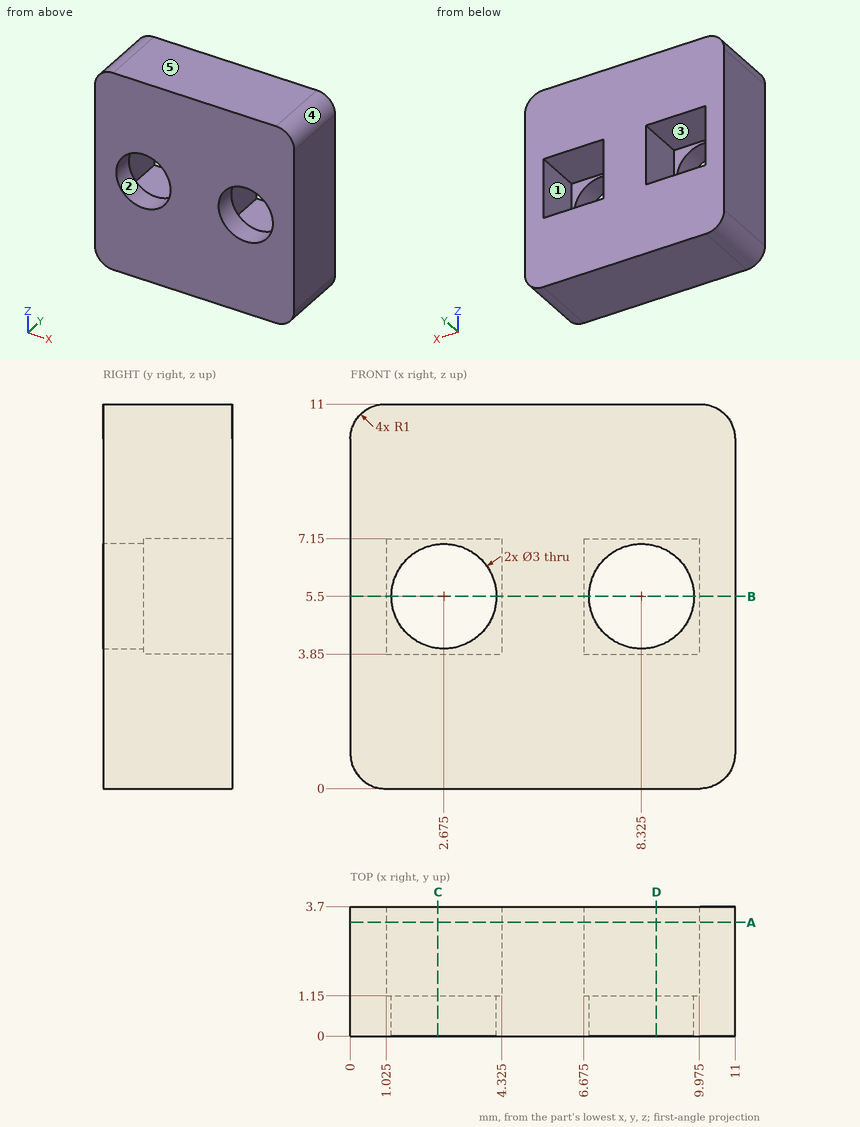
Drawing for the job (mm, zero at the part's lowest x, y, z). A direction names the side the tool comes from. Give positions to 0.01 mm unless a question says otherwise; leave off trailing zeros. Order: outer loops, then holes, each group sorted by start corner. A loop starts at its lowest first (then second) coordinate and runs counter-clockwise, first axis right, second up. Notation, with made-up numbers: M 73.5,-15.75 L 77.5,-15.75 A30 ccw 77.5,17.25 Z; hole C 77.5,57.25 d4. An arc over 180 degrees is marked long. Use a Markdown table: item, result. Add a question column.
(1) Saw through at D-D, the plane x = 8.75. Give the cut face in (y, z).
(2) Saw through at B-B, the plane z = 5.5. Give the cut face in (x, y) (3 decimals), and give its area (3 significant figures).
(3) 3-axis set-ups, long thin cutter, end or side, ignore diameter. For the marked faces 1 and 2: which of +Z, -Z, +X, -X, +Y, -Y reach the whole face in a straight line?
(4) Mould opens along X. For the marked faces 3, 4 and 5 say: +X half, -X half, draft (parallel to the pull), parting line (faces both ways), or undercut.
(5) Probe line 1 along X through (y, z) = (3, 4.25) (3 decimals); line 2 along X through (y, z) = (0.55, 5.5) (3 decimals); line 3 along Z through (x, y) = (4, 1.95). List the from-to ranges inside material, lowest first. Write a range as [from, to].
(6) Saw through at A-A, the plane y = 3.25. Give the cut face in (x, z) (3 decimals).
(7) Saw through at C-C, the plane x = 2.5. Give the cut face in (y, z).
Answer key:
| question | item | result |
|---|---|---|
| 1 | outline | M 0,0 L 3.7,0 L 3.7,3.85 L 1.15,3.85 L 1.15,4.06 L 0,4.06 Z; M 0,6.94 L 1.15,6.94 L 1.15,7.15 L 3.7,7.15 L 3.7,11 L 0,11 Z |
| 2 | outline | M 0,0 L 1.175,0 L 1.175,1.15 L 1.025,1.15 L 1.025,3.7 L 0,3.7 Z; M 4.175,0 L 6.825,0 L 6.825,1.15 L 6.675,1.15 L 6.675,3.7 L 4.325,3.7 L 4.325,1.15 L 4.175,1.15 Z; M 9.825,0 L 11,0 L 11,3.7 L 9.975,3.7 L 9.975,1.15 L 9.825,1.15 Z |
| 2 | area | 17.0 mm^2 |
| 3 | face 1 | +Y |
| 3 | face 2 | +Y, -Y |
| 4 | face 3 | undercut |
| 4 | face 4 | +X half |
| 4 | face 5 | draft |
| 5 | line 1 | [0, 1.025], [4.325, 6.675], [9.975, 11] |
| 5 | line 2 | [0, 1.175], [4.175, 6.825], [9.825, 11] |
| 5 | line 3 | [0, 3.85], [7.15, 11] |
| 6 | outline | M 0,1 A1 ccw 1,0 L 10,0 A1 ccw 11,1 L 11,10 A1 ccw 10,11 L 1,11 A1 ccw 0,10 Z; hole M 1.025,3.85 L 4.325,3.85 L 4.325,7.15 L 1.025,7.15 Z; hole M 6.675,3.85 L 9.975,3.85 L 9.975,7.15 L 6.675,7.15 Z |
| 7 | outline | M 0,0 L 3.7,0 L 3.7,3.85 L 1.15,3.85 L 1.15,4.01 L 0,4.01 Z; M 0,6.99 L 1.15,6.99 L 1.15,7.15 L 3.7,7.15 L 3.7,11 L 0,11 Z |
